```python
from build123d import *

# Parameters (mm, degrees)
SKETCH1_R           = 2.0701
BOSS_EXTRUDE1_DEPTH = 2.286


with BuildPart() as part:
    # Sketch1 → Boss-Extrude1 (new body)
    with BuildSketch(Plane.XY.offset(2.286)):
        with BuildLine():
            Line((17.5895, -24.966646366), (52.272335755, -44.990790925))
            Line((52.272335755, -44.990790925), (54.357769614, -45.549581243))
            Line((54.357769614, -45.549581243), (65.735657525, -25.842501298))
            Line((65.735657525, -25.842501298), (66.294447843, -23.757067439))
            Line((66.294447843, -23.757067439), (5.451427483, 11.370666744))
            Line((5.451427483, 11.370666744), (3.365993624, 11.929457063))
            Line((3.365993624, 11.929457063), (-12.014209682, 3.049692544))
            Line((-12.014209682, 3.049692544), (-12.573, 0.964258685))
            Line((-12.573, 0.964258685), (-12.573, -69.291209682))
            Line((-12.573, -69.291209682), (-10.487566141, -69.85))
            Line((-10.487566141, -69.85), (12.268209682, -69.85))
            Line((12.268209682, -69.85), (12.827, -67.764566141))
            Line((12.827, -67.764566141), (12.827, -27.716277023))
            ThreePointArc((12.827, -27.716277023), (14.4145, -24.966646366), (17.5895, -24.966646366))
        make_face()
        with Locations((54.99261314, -31.75)):
            Circle(SKETCH1_R, mode=Mode.SUBTRACT)
        with Locations((32.995567884, -19.05)):
            Circle(SKETCH1_R, mode=Mode.SUBTRACT)
        with Locations((0, -50.8)):
            Circle(SKETCH1_R, mode=Mode.SUBTRACT)
        with Locations((0, -25.4)):
            Circle(SKETCH1_R, mode=Mode.SUBTRACT)
        with Locations((10.998522628, -6.35)):
            Circle(SKETCH1_R, mode=Mode.SUBTRACT)
        Circle(SKETCH1_R, mode=Mode.SUBTRACT)
        with Locations((0, -12.7)):
            Circle(SKETCH1_R, mode=Mode.SUBTRACT)
        with Locations((0, -38.1)):
            Circle(SKETCH1_R, mode=Mode.SUBTRACT)
        with Locations((21.997045256, -12.7)):
            Circle(SKETCH1_R, mode=Mode.SUBTRACT)
        with Locations((43.994090512, -25.4)):
            Circle(SKETCH1_R, mode=Mode.SUBTRACT)
        with Locations((0, -63.5)):
            Circle(SKETCH1_R, mode=Mode.SUBTRACT)
    extrude(amount=-BOSS_EXTRUDE1_DEPTH)


solid = part.part
```
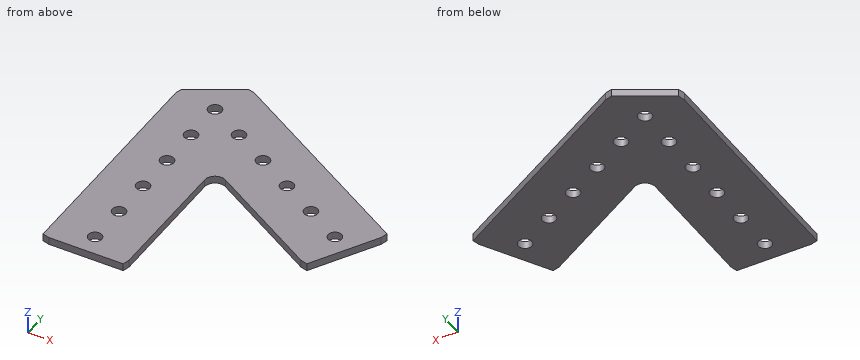
Source: CAD feature listing. Evaluate the final solid. Frame: model axes, mm. Coordinates: 2 decimals unless noted, no trailing zeros. Loops run counter-clockwise (first coordinate to the right, second up) from the corner with the lowest first, then second, coordinate; pieces in that order, holes last. Notation, with made-up numbers: M 73.5,81 L 125.5,81 A11 ccw 125.5,94 Z; hole C 1,-13 d10. An arc over 180 degrees is marked long. Put each result on its own line as item: value. Start each with the question number.
1) Cut plane C-C on x = 0. Return the cut outline in (y, z), then the cut area to 3 significant figures.
2) Cut plane A-A on z = 0.45. Give the number of separate pieces and of enclosed holes in the cut face, then the cut area to 3 significant figures.
3) Contact query for flat-ended pins moving along their axis: pin 1 Ø5 at (x, y) = (22, -12.7) entering from +Z; pin 2 Ø3.5 at (x, y) = (0, -12.7) entering from +Z (3 decimals). Output: stop coordinate, or through.
4) Cut plane D-D on y = -12.7. Return the cut outline in (x, z).
5) Cut plane B-B on y = -63.5. Return the cut outline in (x, z), then the cut area to 3 significant figures.
6) Ray query, L1, parallel to Y at x = 32, z = 1; L2, parallel to X at y = -34.5, z = 2.2; L3, parallel to X at y = -6, z = 1.8. Return the intervals inside material, ascending. Write a range as from..to.
The answers:
1. outline: M -69.85,0 L -65.57,0 L -65.57,2.29 L -69.85,2.29 Z; M -61.43,0 L -52.87,0 L -52.87,2.29 L -61.43,2.29 Z; M -48.73,0 L -40.17,0 L -40.17,2.29 L -48.73,2.29 Z; M -36.03,0 L -27.47,0 L -27.47,2.29 L -36.03,2.29 Z; M -23.33,0 L -14.77,0 L -14.77,2.29 L -23.33,2.29 Z; M -10.63,0 L -2.07,0 L -2.07,2.29 L -10.63,2.29 Z; M 2.07,0 L 9.99,0 L 9.99,2.29 L 2.07,2.29 Z
1. area: 126 mm²
2. separate pieces: 1
2. enclosed holes: 11
2. area: 3,240 mm²
3. pin 1: stops at z = 2.29
3. pin 2: passes through
4. outline: M -12.57,0 L -2.07,0 L -2.07,2.29 L -12.57,2.29 Z; M 2.07,0 L 19.93,0 L 19.93,2.29 L 2.07,2.29 Z; M 24.07,0 L 47.14,0 L 47.14,2.29 L 24.07,2.29 Z
5. outline: M -12.57,0 L -2.07,0 L -2.07,2.29 L -12.57,2.29 Z; M 2.07,0 L 12.83,0 L 12.83,2.29 L 2.07,2.29 Z
5. area: 48.6 mm²
6. L1: y = -33.29..-20.86, -17.24..-3.96
6. L2: x = -12.57..12.83, 34.1..60.74
6. L3: x = -12.57..8.96, 13.04..35.54
